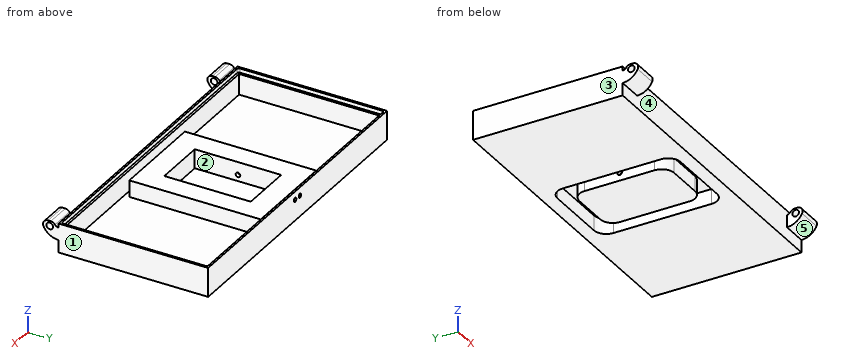
from build123d import *

# Parameters (mm, degrees)
SKETCH1_W                      = 370
SKETCH1_H                      = 180
BOSS_EXTRUDE1_DEPTH            = 35
SKETCH2_W                      = 365.5
SKETCH2_H                      = 175.5
CUT_EXTRUDE1_DEPTH             = 5
SKETCH3_W                      = 360
SKETCH3_H                      = 170
CUT_EXTRUDE2_DEPTH             = 25
SKETCH4_W                      = 115
SKETCH4_H                      = 20
BOSS_EXTRUDE2_DEPTH            = 170
SKETCH5_W                      = 105
SKETCH5_H                      = 148
CUT_EXTRUDE3_DEPTH             = 18
SKETCH6_W                      = 73
SKETCH6_H                      = 114
BOSS_EXTRUDE3_DEPTH            = 18
F_15_0_15_DIAMETER_HOLE1_D     = 5.5
F_15_0_15_DIAMETER_HOLE1_DEPTH = 11
FILLET1_R                      = 2.5
FILLET2_R                      = 15
SKETCH11_W                     = 30
SKETCH11_H                     = 15
REVOLVE1_ANGLE                 = 90
SKETCH12_R                     = 4
CUT_EXTRUDE4_DEPTH             = 371
FILLET4_R                      = 6
FILLET5_R                      = 6
SKETCH13_W                     = 63
SKETCH13_H                     = 104
CUT_EXTRUDE5_DEPTH             = 23
CUT_EXTRUDE6_START             = -20
SKETCH14_W                     = 115
SKETCH14_H                     = 6
CUT_EXTRUDE6_DEPTH             = 20
CUT_EXTRUDE7_START             = -20
SKETCH15_W                     = 115
SKETCH15_H                     = 6
CUT_EXTRUDE7_DEPTH             = 20
CUT_EXTRUDE8_REACH             = 200.649
SKETCH17_R                     = 2.5
SKETCH18_R                     = 2.75
CUT_EXTRUDE9_DEPTH             = 10


with BuildPart() as part:
    # Sketch1 → Boss-Extrude1 (new body)
    with BuildSketch(Plane.XY.offset(35)):
        with Locations((185, 90)):
            Rectangle(SKETCH1_W, SKETCH1_H)
    extrude(amount=-BOSS_EXTRUDE1_DEPTH)

    # Sketch2 → Cut-Extrude1 (cut)
    with BuildSketch(Plane.XY.offset(35)):
        with Locations((185, 90)):
            Rectangle(SKETCH2_W, SKETCH2_H)
    extrude(amount=-CUT_EXTRUDE1_DEPTH, mode=Mode.SUBTRACT)

    # Sketch3 → Cut-Extrude2 (cut)
    with BuildSketch(Plane.XY.offset(30)):
        with Locations((185, 90)):
            Rectangle(SKETCH3_W, SKETCH3_H)
    extrude(amount=-CUT_EXTRUDE2_DEPTH, mode=Mode.SUBTRACT)

    # Sketch4 → Boss-Extrude2 (add)
    with BuildSketch(Plane(origin=(0, 5, 0), x_dir=(-1, 0, 0), z_dir=(0, 1, 0))):
        with Locations((-185, 15)):
            Rectangle(SKETCH4_W, SKETCH4_H)
    extrude(amount=BOSS_EXTRUDE2_DEPTH)

    # Sketch5 → Cut-Extrude3 (cut)
    with BuildSketch(Plane(origin=(0, 0, 0), x_dir=(-1, 0, 0), z_dir=(0, 0, -1))):
        with Locations((-185, 90)):
            Rectangle(SKETCH5_W, SKETCH5_H)
    extrude(amount=-CUT_EXTRUDE3_DEPTH, mode=Mode.SUBTRACT)

    # Sketch6 → Boss-Extrude3 (add)
    with BuildSketch(Plane(origin=(0, 0, 18), x_dir=(-1, 0, 0), z_dir=(0, 0, -1))):
        with Locations((-185, 90)):
            Rectangle(SKETCH6_W, SKETCH6_H)
    extrude(amount=BOSS_EXTRUDE3_DEPTH)

    # Ø15.0 (15) Diameter Hole1
    with Locations(Plane.ZY.offset(-148.5)):
        with Locations((9.5, 90)):
            Hole(F_15_0_15_DIAMETER_HOLE1_D / 2, depth=F_15_0_15_DIAMETER_HOLE1_DEPTH)

    # Fillet1
    fillet1_edges = [part.edges().sort_by_distance(p)[0] for p in [
        (2.25, 177.75, 32.5),
        (367.75, 177.75, 32.5),
        (367.75, 2.25, 32.5),
        (2.25, 2.25, 32.5),
    ]]
    fillet(fillet1_edges, radius=FILLET1_R)

    # Fillet2
    fillet2_edges = [part.edges().sort_by_distance(p)[0] for p in [
        (132.5, 16, 9),
        (237.5, 16, 9),
        (237.5, 164, 9),
        (132.5, 164, 9),
        (148.5, 147, 9),
        (221.5, 147, 9),
        (221.5, 33, 9),
        (148.5, 33, 9),
    ]]
    fillet(fillet2_edges, radius=FILLET2_R)

    # Sketch11 → Revolve1 (revolve)
    with BuildSketch(Plane.XY.offset(35)):
        with Locations((355, -12.5)):
            Rectangle(SKETCH11_W, SKETCH11_H)
        with Locations((15, -12.5)):
            Rectangle(SKETCH11_W, SKETCH11_H)
    revolve(axis=Axis((0, 0, 35), (1, 0, 0)), revolution_arc=REVOLVE1_ANGLE)

    # Sketch12 → Cut-Extrude4 (cut, through all)
    with BuildSketch(Plane(origin=(370, 0, 0), x_dir=(0, 0, -1), z_dir=(1, 0, 0))):
        with Locations((-29, -10.5)):
            Circle(SKETCH12_R)
    extrude(amount=-CUT_EXTRUDE4_DEPTH, mode=Mode.SUBTRACT)

    # Fillet4
    fillet4_edges = [part.edges().sort_by_distance(p)[0] for p in [
        (355, -20, 35),
        (15, -20, 35),
    ]]
    fillet(fillet4_edges, radius=FILLET4_R)

    # Fillet5
    fillet5_edges = [part.edges().sort_by_distance(p)[0] for p in [
        (355, -5, 35),
        (15, -5, 35),
    ]]
    fillet(fillet5_edges, radius=FILLET5_R)

    # Sketch13 → Cut-Extrude5 (cut)
    with BuildSketch(Plane.XY.offset(25)):
        with Locations((185, 90)):
            Rectangle(SKETCH13_W, SKETCH13_H)
    extrude(amount=-CUT_EXTRUDE5_DEPTH, mode=Mode.SUBTRACT)

    # Sketch14 → Cut-Extrude6 (cut)
    with BuildSketch(Plane.XY.offset(25).offset(CUT_EXTRUDE6_START)):
        with Locations((185, 172)):
            Rectangle(SKETCH14_W, SKETCH14_H)
    extrude(amount=CUT_EXTRUDE6_DEPTH, mode=Mode.SUBTRACT)

    # Sketch15 → Cut-Extrude7 (cut)
    with BuildSketch(Plane.XY.offset(25).offset(CUT_EXTRUDE7_START)):
        with Locations((185, 8)):
            Rectangle(SKETCH15_W, SKETCH15_H)
    extrude(amount=CUT_EXTRUDE7_DEPTH, mode=Mode.SUBTRACT)

    # Sketch17 → Cut-Extrude8 (cut, up to next)
    with BuildSketch(Plane(origin=(0, 180, 0), x_dir=(1, 0, 0), z_dir=(0, 1, 0)), mode=Mode.PRIVATE) as cut_extrude8_sk1:
        with Locations((180, -25)):
            Circle(SKETCH17_R)
    cut_extrude8_tool1 = extrude(cut_extrude8_sk1.sketch, amount=-CUT_EXTRUDE8_REACH, mode=Mode.PRIVATE) & part.part
    add(cut_extrude8_tool1.solids().sort_by_distance((180, 180, 25))[0], mode=Mode.SUBTRACT)
    # Sketch17 → Cut-Extrude8 (cut, up to next)
    with BuildSketch(Plane(origin=(0, 180, 0), x_dir=(1, 0, 0), z_dir=(0, 1, 0)), mode=Mode.PRIVATE) as cut_extrude8_sk2:
        with Locations((190, -25)):
            Circle(SKETCH17_R)
    cut_extrude8_tool2 = extrude(cut_extrude8_sk2.sketch, amount=-CUT_EXTRUDE8_REACH, mode=Mode.PRIVATE) & part.part
    add(cut_extrude8_tool2.solids().sort_by_distance((190, 180, 25))[0], mode=Mode.SUBTRACT)

    # Sketch18 → Cut-Extrude9 (cut)
    with BuildSketch(Plane(origin=(221.5, 0, 0), x_dir=(0, 0, -1), z_dir=(1, 0, 0))):
        with Locations((-9.5, 90)):
            Circle(SKETCH18_R)
    extrude(amount=-CUT_EXTRUDE9_DEPTH, mode=Mode.SUBTRACT)


solid = part.part
For this review, take the finished solid that the model builds, in its own axes (mm). Face numbers are marked on the shaded views. A direction names the side the tool comes from. Round coordinates to 2 decimals unless told otherwise and drop trailing zeros. Write each loop counter-clockwise with the first axis right and the second up, starting at its lowest first coordinate (ties: lowest second). Pieces come first, ordered by that corner, then holes. Notation, with made-up numbers: (-29, 26.5) -> (10, 26.5) arc R25 cw to (10, 43.5) -> close; hole circle Ø3 at (75.5, 81.25). An arc over 180 degrees is marked (long way). Put each result on its own line as item: value.
Q1. Clearance check with flat-ended pins moving along their axes: pin 1 Ø2 at (y, z) = (61, 21) entering from -X; pin 2 Ø19 at (x, y) = (190, 74) entering from +Z; pin 3 Ø10 at (x, y) = (229.5, 78) entering from +Z; pin 4 Ø6 at (x, z) = (194.5, 14) entering from -Y. State where each tip first meets the part, or that it passes through.
Determined:
pin 1: stops at x = 0
pin 2: stops at z = 2
pin 3: stops at z = 25
pin 4: stops at y = 0
Q2. Consider section D-D on y = 23. State the section outline as (x, z) points.
Determined:
outline: (0, 0) -> (134.81, 0) -> (134.81, 18) -> (235.19, 18) -> (235.19, 0) -> (370, 0) -> (370, 35) -> (367.75, 35) -> (367.75, 30) -> (365, 30) -> (365, 5) -> (242.5, 5) -> (242.5, 25) -> (127.5, 25) -> (127.5, 5) -> (5, 5) -> (5, 30) -> (2.25, 30) -> (2.25, 35) -> (0, 35) -> close
Q3. To check wall thickness, follow L1, parallel to Y at x = 12.75, z = 29; L2, parallel to X at y = 155, z = 19.5; L3, parallel to X at y = 88.5, z = 4.5. State the ranges of each line that lie inside material, in increasing order. Write a range as [from, to].
Determined:
L1: y = [-18.65, -14.5], [-6.5, 5], [175, 180]
L2: x = [0, 5], [127.5, 242.5], [365, 370]
L3: x = [0, 132.5], [148.5, 153.5], [216.5, 221.5], [237.5, 370]
Q4. Consider section C-C on y = 137.5. State the section outline as (x, z) points.
Determined:
outline: (0, 0) -> (132.5, 0) -> (132.5, 18) -> (149.54, 18) -> (149.54, 0) -> (220.46, 0) -> (220.46, 18) -> (237.5, 18) -> (237.5, 0) -> (370, 0) -> (370, 35) -> (367.75, 35) -> (367.75, 30) -> (365, 30) -> (365, 5) -> (242.5, 5) -> (242.5, 25) -> (216.5, 25) -> (216.5, 2) -> (153.5, 2) -> (153.5, 25) -> (127.5, 25) -> (127.5, 5) -> (5, 5) -> (5, 30) -> (2.25, 30) -> (2.25, 35) -> (0, 35) -> close
Q5. The part is to be moulded in two halves that separate along X. For the marked faces 3, 4 and 5, say which applies: released by +X, released by -X, zero draft, split by the parting line, or undercut.
Determined:
face 3: released by -X
face 4: undercut
face 5: zero draft
Q6. Consider section A-A on y = 73.5. State the section outline as (x, z) points.
Determined:
outline: (0, 0) -> (132.5, 0) -> (132.5, 18) -> (148.5, 18) -> (148.5, 0) -> (221.5, 0) -> (221.5, 18) -> (237.5, 18) -> (237.5, 0) -> (370, 0) -> (370, 35) -> (367.75, 35) -> (367.75, 30) -> (365, 30) -> (365, 5) -> (242.5, 5) -> (242.5, 25) -> (216.5, 25) -> (216.5, 2) -> (153.5, 2) -> (153.5, 25) -> (127.5, 25) -> (127.5, 5) -> (5, 5) -> (5, 30) -> (2.25, 30) -> (2.25, 35) -> (0, 35) -> close
Q7. Machinability: for the marked faces 1 and 2, which of the approach directions +Z, -Z, +X, -X, +Y, -Y give a long, thin tool a straight path to every point of the face, cutting with its end or side? Answer none if there is none.
Determined:
face 1: +Z, -Z, +X, +Y, -Y
face 2: +Z
Q8. Consider section B-B on x = 99. State the section outline as (y, z) points, and give its area (3 significant figures).
Determined:
outline: (0, 0) -> (180, 0) -> (180, 35) -> (177.75, 35) -> (177.75, 30) -> (175, 30) -> (175, 5) -> (5, 5) -> (5, 30) -> (2.25, 30) -> (2.25, 35) -> (0, 35) -> close
area: 1,170 mm^2
